```python
from build123d import *

# Parameters (mm, degrees)
F1_DEPTH = 54
F2_W     = 12
F2_H     = 30
F3_DEPTH = 17


with BuildPart() as f1:
    # F0 (on Top) → F1 (new body)
    with BuildSketch(Plane.XY):
        Polygon((17, 15), (-17, 15), (-17, -15), (-8, -15), (-8, -7), (0, -7), (8, -7), (8, -15), (17, -15), align=None)
    extrude(amount=F1_DEPTH)

    # F2 (on face) → F3 (cut)
    with BuildSketch(Plane(origin=(-17, 0, 0), x_dir=(0, -1, 0), z_dir=(-1, 0, 0))):
        with Locations((-9, 27)):
            Rectangle(F2_W, F2_H)
    extrude(amount=-F3_DEPTH, mode=Mode.SUBTRACT)


solid = f1.part
```
Could you check a few things on this model? Use its own coordinates, in mm. A direction names the side the tool comes from. Give positions to 0.01 mm unless a question says otherwise; leave off trailing zeros. Order: outer loops, then holes, each group sorted by start corner. A loop starts at its lowest first (then second) coordinate and runs counter-clockwise, first axis right, second up.
Q1. Suppose I cut it at A-A, the plane z = 44.5. Write out the boundary of the cut face in (x, y).
Q2. For faces 4 (the flat face through (8, -11, 27)), 5 (the flat face through (-13, -15, 27)), 6 (the flat face through (0, 9, 27)), which set-ups out of +Z, -Z, +X, -X, +Y, -Y let a thin tool reach every point of the face, with its end or its side?
Q3. Suppose I cut it at C-C, the plane z = 31. Write out the boundary of the cut face in (x, y).
Q4. If I drill on line 1 along Z through (x, y) = (-11, 5.25); line 2 along X through (y, z) = (5.25, 18); line 3 along Y through (x, z) = (-5, 29.5), over which ranges is the centre line in solid material (lowest first)?
Q5. Suppose I cut it at D-D, the plane x = 3. Write out the boundary of the cut face in (y, z).
Q6. Suppose I cut it at B-B, the plane x = -3. Write out the boundary of the cut face in (y, z).
Q7. I'm going to push flat-ended pins straight in: P1, Ø6, axis at x = 12.5, y = 6.5, coming from the -Z side; P2, Ø5, axis at x = 3, z = 22.5, coming from the -Y side; P3, Ø3.5, axis at y = 8, z = 26.5, coming from the -X side; P4, Ø8.5, axis at x = -7.5, z = 23, coming from the +Y side. Where does each tip first touch, or does it pass through?
Q8. We'd pull the mould along Z, two halves only. Please class faces 1 (the flat face through (0, 0, 54)), 2 (the flat face through (-17, -3, 27)), 3 (the flat face through (-9, 3, 27)): +Z half, -Z half, draft (parallel to the pull), parting line (faces both ways), or undercut.
Solution:
1. outline: (-17, -15) - (-8, -15) - (-8, -7) - (8, -7) - (8, -15) - (17, -15) - (17, 15) - (-17, 15) - close
2. face 4: +Z, -Z, -Y
2. face 5: +Z, -Z, +X, -X, -Y
2. face 6: -X, +Y
3. outline: (-17, -15) - (-8, -15) - (-8, -7) - (8, -7) - (8, -15) - (17, -15) - (17, 15) - (0, 15) - (0, 3) - (-17, 3) - close
4. line 1: z = 0 to 12, 42 to 54
4. line 2: x = 0 to 17
4. line 3: y = -7 to 3
5. outline: (-7, 0) - (15, 0) - (15, 54) - (-7, 54) - close
6. outline: (-7, 0) - (15, 0) - (15, 12) - (3, 12) - (3, 42) - (15, 42) - (15, 54) - (-7, 54) - close
7. P1: stops at z = 0
7. P2: stops at y = -7
7. P3: stops at x = 0
7. P4: stops at y = 3
8. face 1: +Z half
8. face 2: draft
8. face 3: undercut
